Part model, mm, in its own coordinate system. Face numbers are marked on the shaded views. A direction names the side the tool comes from. Round coordinates to 2 decimals unless told otherwise and drop trailing zeros. Write each loop counter-clockwise with the first axis right and the second up, starting at its lowest first coordinate (ties: lowest second). Pieces come first, ordered by that corner, then holes.
1) Saw through at C-C on z = 12.5. Write the cut outline in (x, y).
2) Saw through at D-D on y = -3. Write the cut outline in (x, z), and give its area (3 significant figures).
3) Saw through at A-A on x = 65. Write the cut outline in (y, z).
4) Saw through at B-B on y = 42. Write the cut outline in (x, z), and give its area (3 significant figures).
5) Pull direction X, two halves, no side cores. Call the marked faces 3, 4, 5 and 6: +X half, -X half, draft (parallel to the pull), parting line (faces both ways), or undercut.
6) Which spindle directions (+Z, -Z, +X, -X, +Y, -Y) get a long thin tool onto all of the face, cutting with end or side? Do the marked faces 1 and 2. Say none if no direction does.
7) Drill centre lines: L1, parallel to Y at x = 99, z = 55; L2, parallel to X at y = 42, z = 37; L3, parallel to Y at x = 88.5, z = 56.5. Where is each one in solid material? Low to high.
8) Flat gauge pin, fed straight in: pin 1 (3 mm diameter, centred on x = 40.5, y = -4, fed in from +Z). Where does the tip first touch, or does it go through?
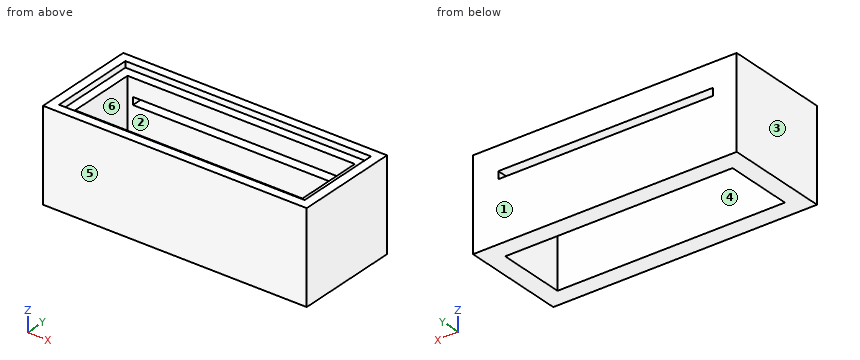
```python
from build123d import *

# Parameters (mm, degrees)
PAD_DEPTH       = 60
PAD001_DEPTH    = 60
PAD004_DEPTH    = 60
PAD006_DEPTH    = 60
SKETCH008_W     = 162
SKETCH008_H     = 57
POCKET_DEPTH    = 4
SKETCH011_W     = 141.774313
SKETCH011_H     = 4.907572
POCKET001_DEPTH = 12


with BuildPart() as part:
    # Sketch → Pad (new body)
    with BuildSketch(Plane.XY):
        Polygon((162, -12), (150, 0), (0, 0), (-12, -12), align=None)
    extrude(amount=PAD_DEPTH)

    # Sketch001 → Pad001 (join)
    with BuildSketch(Plane.XY):
        Polygon((0, 45), (0, 0), (-12, -12), (-12, 57), align=None)
    extrude(amount=PAD001_DEPTH)

    # Sketch004 → Pad004 (join)
    with BuildSketch(Plane.XY):
        Polygon((150, 0), (162, -12), (162, 57), (150, 45), align=None)
    extrude(amount=PAD004_DEPTH)

    # Sketch007 → Pad006 (join)
    with BuildSketch(Plane.XY):
        Polygon((-12, 57), (162, 57), (150, 45), (0, 45), align=None)
    extrude(amount=PAD006_DEPTH)

    # Sketch008 (on Face13 of Pad006) → Pocket (cut)
    with BuildSketch(Plane.XY.offset(60)):
        with Locations((75, 22.5)):
            Rectangle(SKETCH008_W, SKETCH008_H)
    extrude(amount=-POCKET_DEPTH, mode=Mode.SUBTRACT)

    # Sketch011 (on Face6 of Pad006) → Pocket001 (cut)
    with BuildSketch(Plane(origin=(0, 57, 0), x_dir=(-1, 0, 0), z_dir=(0, 1, 0))):
        with Locations((-74.422004, 41.981674)):
            Rectangle(SKETCH011_W, SKETCH011_H)
    extrude(amount=-POCKET001_DEPTH, mode=Mode.SUBTRACT)


solid = part.part
```
Completed:
1. outline: (-12, -12) - (162, -12) - (162, 57) - (-12, 57) - close; hole (0, 0) - (150, 0) - (150, 45) - (0, 45) - close
2. outline: (-12, 0) - (162, 0) - (162, 60) - (156, 60) - (156, 56) - (-6, 56) - (-6, 60) - (-12, 60) - close
2. area: 9,790 mm2
3. outline: (-12, 0) - (0, 0) - (0, 56) - (-6, 56) - (-6, 60) - (-12, 60) - close; (45, 0) - (57, 0) - (57, 39.53) - (45, 39.53) - close; (45, 44.44) - (57, 44.44) - (57, 60) - (51, 60) - (51, 56) - (45, 56) - close
4. outline: (-12, 0) - (0, 0) - (0, 56) - (-6, 56) - (-6, 60) - (-12, 60) - close; (150, 0) - (162, 0) - (162, 60) - (156, 60) - (156, 56) - (150, 56) - close
4. area: 1,390 mm2
5. face 3: -X half
5. face 4: undercut
5. face 5: draft
5. face 6: undercut
6. face 1: +Z, -Z, +X, -X, +Y
6. face 2: +Z, -Z
7. L1: y = -12 to 0, 45 to 57
7. L2: x = -12 to 0, 150 to 162
7. L3: y = -12 to -6, 51 to 57
8. pin 1: stops at z = 56
